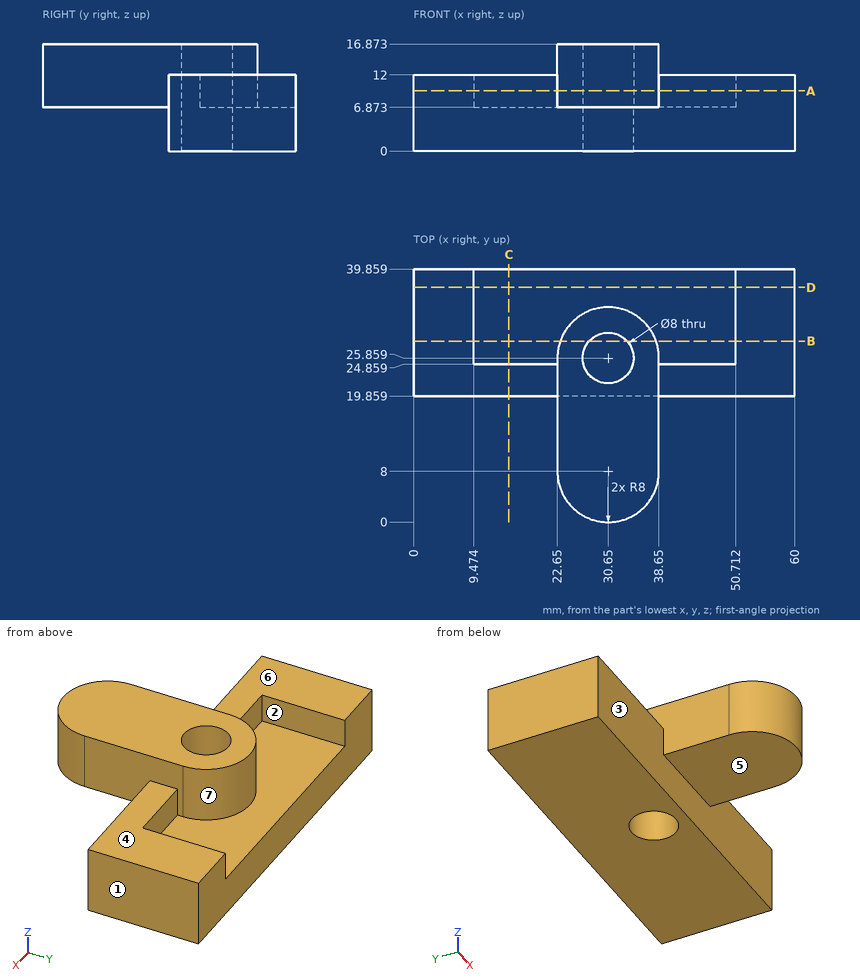
Input: dimensioned drawing with shaded views. Units: mm. Origin: part minimum x, y, z. A direction names the side the tool comes from. Coordinates: 2 decimals unless noted, no trailing zeros. Order: outer loops, then holes, each group sorted by start corner. A loop starts at its lowest first (then second) coordinate and runs counter-clockwise, first axis right, second up. Notation, with made-up numbers: (-10, 40) - (32, 40) arc R20 cw to (32, 58) - close; hole circle Ø9 at (-33, 75). An arc over 180 degrees is marked (long way). Return JSON: item names as keys, results as strings. Group by question number.
1. Cut plane C-C (x = 15). Output: boundary loops of the cut face in (y, z).
2. Material intervals for line 1 along Y through (x, z) = (30.5, 12.5); line 2 along Y through (x, z) = (13.5, 11.25); line 3 along Z through (x, y) = (24, 12.5), sorted ascending. Write a range as [from, to].
3. Set-up query: the marked faces 4, 5, 6 and 7. Return all of +Z, -Z, +X, -X, +Y, -Y with unobstructed straight access to the full face (end or side cutting, diameter ignored); none if empty.
4. Cut plane B-B (y = 28.5). Output: boundary loops of the cut face in (x, z), plus the area to 3 significant figures.
5. Cut plane D-D (y = 37). Output: boundary loops of the cut face in (x, z).
6. Cut plane A-A (z = 9.5). Output: boundary loops of the cut face in (x, y).
7. Pull-direction query (X, two-part tool) for the marked faces 1, 2 and 3; classes: pulls with the +X half, pulls with the -X half, needs draft (parallel to the pull), parting line crosses it, or undercut.
8. Pin query (flat end, axial travel): pin 1 (3 mm diameter, centred on x = 31, y = 8.5, fed in from -Z); pin 2 (4 mm diameter, centred on x = 45, z = 10.5, fed in from +Y); pin 3 (2 mm diameter, centred on x = 24, z = 5.5, fed in from -Y); pin 4 (6.5 mm diameter, centred on x = 30.65, y = 25.86, fed in from -Z). Return the tip coordinate at first contact, or that it passes through.
Resolved:
{
 "1": {"outline": "(19.86, 0) - (39.86, 0) - (39.86, 6.87) - (24.86, 6.87) - (24.86, 12) - (19.86, 12) - close"},
 "2": {"line 1": "y = [0, 21.86], [29.86, 33.86]", "line 2": "y = [19.86, 24.86]", "line 3": "z = [6.87, 16.87]"},
 "3": {"face 4": "+Z, +X, +Y, -Y", "face 5": "-Z, +X, -X, -Y", "face 6": "+Z, -X, +Y, -Y", "face 7": "+Z, +Y"},
 "4": {"outline": "(0, 0) - (27.65, 0) - (27.65, 16.87) - (23.1, 16.87) - (23.1, 6.87) - (9.47, 6.87) - (9.47, 12) - (0, 12) - close; (33.65, 0) - (60, 0) - (60, 12) - (50.71, 12) - (50.71, 6.87) - (38.2, 6.87) - (38.2, 16.87) - (33.65, 16.87) - close", "area": "558 mm²"},
 "5": {"outline": "(0, 0) - (60, 0) - (60, 12) - (50.71, 12) - (50.71, 6.87) - (9.47, 6.87) - (9.47, 12) - (0, 12) - close"},
 "6": {"outline": "(0, 19.86) - (22.65, 19.86) - (22.65, 8) arc R8 ccw to (38.65, 8) - (38.65, 19.86) - (60, 19.86) - (60, 39.86) - (50.71, 39.86) - (50.71, 24.86) - (38.65, 24.86) - (38.65, 25.86) arc R8 ccw to (22.65, 25.86) - (22.65, 24.86) - (9.47, 24.86) - (9.47, 39.86) - (0, 39.86) - close; hole circle Ø8 at (30.65, 25.86)"},
 "7": {"face 1": "pulls with the +X half", "face 2": "undercut", "face 3": "needs draft"},
 "8": {"pin 1": "stops at z = 6.87", "pin 2": "stops at y = 24.86", "pin 3": "stops at y = 19.86", "pin 4": "passes through"}
}
